Read the model definition and answer for the solid it produces. Units are mm, in the model's axes. Round coordinates to 2 decimals unless told otherwise and drop trailing zeros. Loops run counter-clockwise (first coordinate to the right, second up) from the corner with the lowest first, then second, coordinate; pieces in that order, holes last. Notation, with made-up numbers: M -7.5,72 L 23.5,72 A20 cw 23.5,95 Z; hole C 29,69 d4. An arc over 180 degrees is marked long. Write each question's results on one line, items separated by ' | '.
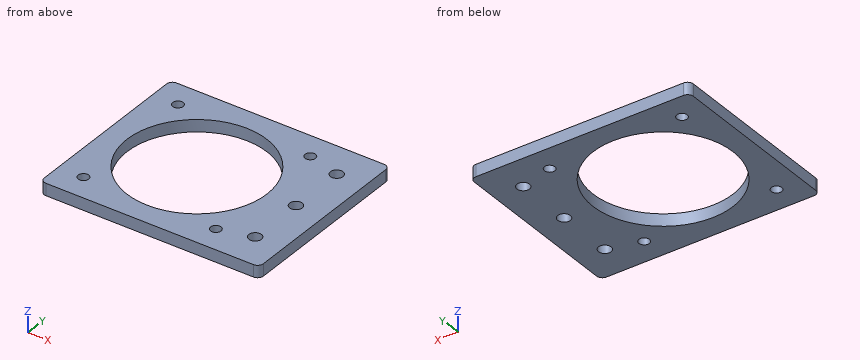
from build123d import *

# Parameters (mm, degrees)
SKETCH1_W                = 115
SKETCH1_H                = 96
BOSS_EXTRUDE1_DEPTH      = 6.35
SKETCH2_R                = 36.75
CUT_EXTRUDE1_DEPTH       = 7.35
FILLET1_R                = 3
M6_CLEARANCE_HOLE1_D     = 6.6
M6_CLEARANCE_HOLE1_DEPTH = 20
M6_CLEARANCE_HOLE1_TIP   = 1.982840043
M5_CLEARANCE_HOLE1_D     = 5.5


with BuildPart() as part:
    # Sketch1 → Boss-Extrude1 (new body)
    with BuildSketch(Plane.XY):
        Rectangle(SKETCH1_W, SKETCH1_H)
    extrude(amount=BOSS_EXTRUDE1_DEPTH)

    # Sketch2 → Cut-Extrude1 (cut, through all)
    with BuildSketch(Plane.XY.offset(6.35)):
        with Locations((-9.5, 0)):
            Circle(SKETCH2_R)
    extrude(amount=-CUT_EXTRUDE1_DEPTH, mode=Mode.SUBTRACT)

    # Fillet1
    fillet1_edges = [part.edges().sort_by_distance(p)[0] for p in [
        (57.5, -48, 3.175),
        (-57.5, -48, 3.175),
        (-57.5, 48, 3.175),
        (57.5, 48, 3.175),
    ]]
    fillet(fillet1_edges, radius=FILLET1_R)

    # M6 Clearance Hole1
    with Locations(Plane.XY.offset(6.35)):
        with Locations((42.5, 30), (42.5, 0), (42.5, -30)):
            Hole(M6_CLEARANCE_HOLE1_D / 2, depth=M6_CLEARANCE_HOLE1_DEPTH)
            with Locations((0, 0, -(M6_CLEARANCE_HOLE1_DEPTH + M6_CLEARANCE_HOLE1_TIP / 2))):  # 118° drill point
                Cone(0, M6_CLEARANCE_HOLE1_D / 2, M6_CLEARANCE_HOLE1_TIP, mode=Mode.SUBTRACT)

    # M5 Clearance Hole1 (through all)
    with Locations(Plane.XY.offset(6.35)):
        with Locations((25.25, -34.75), (-44.25, -34.75), (-44.25, 34.75), (25.25, 34.75)):
            Hole(M5_CLEARANCE_HOLE1_D / 2)


solid = part.part
Item 1: The part is cut by section D-D (x = 42.5). Determine the outline of the cut face in (y, z).
Outcome:
outline: M -48,0 L -33.3,0 L -33.3,6.35 L -48,6.35 Z; M -26.7,0 L -3.3,0 L -3.3,6.35 L -26.7,6.35 Z; M 3.3,0 L 26.7,0 L 26.7,6.35 L 3.3,6.35 Z; M 33.3,0 L 48,0 L 48,6.35 L 33.3,6.35 Z
Item 2: Flat-ended cylindrical pins translate along their axes: pin 1 (5 mm diameter, centred on x = -16.5, y = -33, fed in from -Z); pin 2 (10.5 mm diameter, centred on x = 42.5, y = 0, fed in from -Z). Find the tip coordinate at first contact, or state that the pin passes through.
Outcome:
pin 1: passes through | pin 2: stops at z = 0
Item 3: Straight lines are drawn through the part: line 1 (Y direction, x = 42.5, z = 1.75); line 2 (X direction, y = -30.5, z = 4.75); line 3 (X direction, y = -33, z = 5). For each, find the intervals that lie inside material, in ascending order.
Outcome:
line 1: y = -48 to -33.3, -26.7 to -3.3, 3.3 to 26.7, 33.3 to 48 | line 2: x = -57.5 to -30, 11 to 39.24, 45.76 to 57.5 | line 3: x = -57.5 to -46.37, -42.13 to -25.67, 6.67 to 23.13, 27.37 to 41.13, 43.87 to 57.5
Item 4: The part is cut by section A-A (x = -9.5). Determine the outline of the cut face in (y, z), plus the area to 3 significant figures.
Outcome:
outline: M -48,0 L -36.75,0 L -36.75,6.35 L -48,6.35 Z; M 36.75,0 L 48,0 L 48,6.35 L 36.75,6.35 Z | area: 143 mm2
Item 5: The part is cut by section B-B (z = 4). State how many separate pieces and enclosed holes the cut face has, plus the area to 3 significant figures.
Outcome:
separate pieces: 1 | enclosed holes: 8 | area: 6,590 mm2
Item 6: The part is cut by section C-C (y = 0). Determine the outline of the cut face in (x, z).
Outcome:
outline: M -57.5,0 L -46.25,0 L -46.25,6.35 L -57.5,6.35 Z; M 27.25,0 L 39.2,0 L 39.2,6.35 L 27.25,6.35 Z; M 45.8,0 L 57.5,0 L 57.5,6.35 L 45.8,6.35 Z
